```python
from build123d import *

# Parameters (mm, degrees)
BOSS_EXTRUDE1_DEPTH   = 14
SKETCH2_R             = 2.15
CUT_EXTRUDE1_DEPTH    = 25
CUT_EXTRUDE2_START    = -5.6
SKETCH3_R             = 4.3
CUT_EXTRUDE2_DEPTH    = 19.4
CHAMFER1_SIZE         = 2.1
CHAMFER2_SIZE         = 0.4
CHAMFER2_EDGE_2_SIZE  = 0.4
CHAMFER2_EDGE_3_SIZE2 = 0.4
CHAMFER2_EDGE_3_SIZE  = 0.282842712
CHAMFER2_EDGE_4_SIZE2 = 0.282842712
CHAMFER2_EDGE_4_SIZE  = 0.4
FILLET1_R             = 0.5


with BuildPart() as part:
    # Sketch1 → Boss-Extrude1 (new body)
    with BuildSketch(Plane(origin=(0, 0, 0), x_dir=(1, 0, 0), z_dir=(0, 1, 0))):
        Polygon((0, 0), (33.941125497, 0), (16.970562748, -16.970562748), align=None)
    extrude(amount=BOSS_EXTRUDE1_DEPTH)

    # Sketch2 → Cut-Extrude1 (cut, through all)
    with BuildSketch(Plane(origin=(0, 0, 0), x_dir=(0.707106781, 0, 0.707106781), z_dir=(-0.707106781, 0, 0.707106781))):
        with Locations((14, 7)):
            Circle(SKETCH2_R)
    cut_extrude1 = extrude(amount=-CUT_EXTRUDE1_DEPTH, mode=Mode.SUBTRACT)

    # Sketch3 → Cut-Extrude2 (cut, through all)
    with BuildSketch(Plane(origin=(0, 0, 0), x_dir=(0.707106781, 0, 0.707106781), z_dir=(-0.707106781, 0, 0.707106781)).offset(CUT_EXTRUDE2_START)):
        with Locations((14, 7)):
            Circle(SKETCH3_R)
    cut_extrude2 = extrude(amount=-CUT_EXTRUDE2_DEPTH, mode=Mode.SUBTRACT)

    # Mirror1: Cut-Extrude1, Cut-Extrude2 across plane
    add(cut_extrude1.mirror(Plane(origin=(16.970562748, 0, 0), x_dir=(0, 0, 1), z_dir=(1, 0, 0))), mode=Mode.SUBTRACT)
    add(cut_extrude2.mirror(Plane(origin=(16.970562748, 0, 0), x_dir=(0, 0, 1), z_dir=(1, 0, 0))), mode=Mode.SUBTRACT)

    # Chamfer1
    chamfer1_edges = [part.edges().sort_by_distance(p)[0] for p in [
        (12.339013332, 7, 4.419417382),
        (21.602112165, 7, 4.419417382),
    ]]
    chamfer(chamfer1_edges, length=CHAMFER1_SIZE)

    # Chamfer2
    chamfer2_edges = [part.edges().sort_by_distance(p)[0] for p in [
        (16.970562748, 14, 0),
    ]]
    chamfer(chamfer2_edges, length=CHAMFER2_SIZE)

    # Chamfer2 edge 2
    chamfer2_edge_2_edges = [part.edges().sort_by_distance(p)[0] for p in [
        (16.970562748, 0, 0),
    ]]
    chamfer(chamfer2_edge_2_edges, length=CHAMFER2_EDGE_2_SIZE)

    # Chamfer2 edge 3
    chamfer2_edge_3_edges = [part.edges().sort_by_distance(p)[0] for p in [
        (0, 7, 0),
    ]]
    chamfer(chamfer2_edge_3_edges, length=CHAMFER2_EDGE_3_SIZE, length2=CHAMFER2_EDGE_3_SIZE2)

    # Chamfer2 edge 4
    chamfer2_edge_4_edges = [part.edges().sort_by_distance(p)[0] for p in [
        (33.941125497, 7, 0),
    ]]
    chamfer(chamfer2_edge_4_edges, length=CHAMFER2_EDGE_4_SIZE, length2=CHAMFER2_EDGE_4_SIZE2)

    # Fillet1
    fillet1_edges = [part.edges().sort_by_distance(p)[0] for p in [
        (11.523443743, 3.119120407, 0),
        (22.417681754, 3.119120407, 0),
    ]]
    fillet(fillet1_edges, radius=FILLET1_R)


solid = part.part
```
Source: CAD feature listing. Evaluate the final solid. Frame: model axes, mm. A direction names the side the tool comes from. Round coordinates to 2 decimals unless told otherwise and drop trailing zeros. Loops run counter-clockwise (first coordinate to the right, second up) from the corner with the lowest first, then second, coordinate; pieces in that order, holes last.
1. Section query A-A on y = 12.75. Output: boundary loops of the cut face in (x, z), and give its area (3 significant figures).
2. Mould query, pull axis Y, two halves, no side actions, for faces 3 (the cylindrical face through (23.02, 9.13, 8.48)), 4 (the conical face through (13.21, 4.98, 8.08)), 5 (the flat face through (17, 14, 7)), 6 (the flat face through (9, 5, 9)). Classes: released by +Y, released by -Y, zero draft, split by the parting line, or undercut.
3. Section query C-C on z = 15.25. Output: boundary loops of the cut face in (x, y), and give its area (3 significant figures).
4. Access query for faces 1 (the flat face through (17, 0, 7)), 2 (the conical face through (23.085, 6.9, 5.72)). Directions: +Z, -Z, +X, -X, +Y, -Y. A direction counts if a zero-diameter tool reaches every point of the face in a straight line with its end or side. Return the directions, or none.
5. Contact query for flat-ended pins moving along their axis: pin 1 (8 mm diameter, centred on y = 11.5, z = 6, fed in from +X); pin 2 (1 mm diameter, centred on x = 21.5, y = 2, fed in from +Z); pin 3 (8 mm diameter, centred on x = 10, y = 11.5, fed in from +Z). Output: stop coordinate, or through.
6. Section query B-B on y = 6. Give the number of separate pieces and of enclosed holes in the cut face, and give its area (3 significant figures).
7. Ray query, L1, parallel to Y at x = 19, z = 2.25; L2, parallel to X at y = 6.5, z = 5; L3, parallel to Y at x = 17.5, z = 3.75. Return the intervals inside material, ascending.
Answers below:
1. outline: (0.2, 0.2) - (0.4, 0) - (33.66, 0) - (33.66, 0.28) - (16.97, 16.97) - close
1. area: 288 mm2
2. face 3: undercut
2. face 4: undercut
2. face 5: released by +Y
2. face 6: zero draft
3. outline: (15.25, 0) - (18.69, 0) - (18.69, 14) - (15.25, 14) - close
3. area: 48.2 mm2
4. face 1: +Z, -Z, +X, -X, -Y
4. face 2: none
5. pin 1: stops at x = 31.94
5. pin 2: stops at z = 12.94
5. pin 3: stops at z = 14
6. separate pieces: 3
6. enclosed holes: 0
6. area: 156 mm2
7. L1: y = 0 to 2.82, 11.18 to 14
7. L2: x = 5 to 10.89, 23.06 to 28.94
7. L3: y = 0 to 2.71, 11.29 to 14
